from build123d import *

# Parameters (mm, degrees)
SKETCH1_R           = 4.69
SKETCH1_R_2         = 2.2
BOSS_EXTRUDE3_DEPTH = 30
SKETCH3_R           = 4.14334423
SKETCH3_R_2         = 2.739824148
BOSS_EXTRUDE4_DEPTH = 10
SKETCH4_R           = 2.757198723
SKETCH4_R_2         = 1.67402832
BOSS_EXTRUDE5_DEPTH = 10
SKETCH5_R           = 2.2
SKETCH5_R_2         = 1.417715224
BOSS_EXTRUDE6_DEPTH = 10
FILLET13_R          = 5
FILLET15_R          = 5
FILLET16_R          = 5
FILLET17_R          = 5
FILLET19_R          = 5
FILLET20_R          = 5
FILLET21_R          = 5
BOSS_EXTRUDE7_START = -20
SKETCH6_R           = 7.130132291
BOSS_EXTRUDE7_DEPTH = 5
SKETCH7_R           = 3.768659845
CUT_EXTRUDE1_DEPTH  = 30
FILLET26_R          = 5
FILLET27_R          = 5
FILLET28_R          = 5
FILLET29_R          = 5
FILLET30_R          = 5


with BuildPart() as part:
    # Sketch1 → Boss-Extrude3 (new body)
    with BuildSketch(Plane.XY):
        Circle(SKETCH1_R)
        Circle(SKETCH1_R_2, mode=Mode.SUBTRACT)
    extrude(amount=BOSS_EXTRUDE3_DEPTH)

    # Sketch3 → Boss-Extrude4 (add)
    with BuildSketch(Plane.XY.offset(30)):
        Circle(SKETCH3_R)
        Circle(SKETCH3_R_2, mode=Mode.SUBTRACT)
    extrude(amount=BOSS_EXTRUDE4_DEPTH)

    # Sketch4 → Boss-Extrude5 (add)
    with BuildSketch(Plane.XY.offset(40)):
        Circle(SKETCH4_R)
        Circle(SKETCH4_R_2, mode=Mode.SUBTRACT)
    extrude(amount=BOSS_EXTRUDE5_DEPTH)

    # Sketch5 → Boss-Extrude6 (add)
    with BuildSketch(Plane.XY.offset(50)):
        Circle(SKETCH5_R)
        Circle(SKETCH5_R_2, mode=Mode.SUBTRACT)
    extrude(amount=BOSS_EXTRUDE6_DEPTH)

    # Fillet13
    # the kernel refuses this fillet: 5 mm, written as the material it takes off along each edge
    with BuildSketch(Plane(origin=(0, 0, 50), x_dir=(1, 0, 0), z_dir=(0, -1, 0))) as fillet13_piece_1:
        with BuildLine():
            CenterArc((6.417715224, 1.580327356), FILLET13_R, 180, 18.425147301)
            Line((1.417715224, 1.580327356), (1.317715224, 1.580327356))
            Line((1.317715224, 1.580327356), (1.317715224, 0))
            Line((1.317715224, 0), (1.417715224, -0.1))
            ThreePointArc((1.417715224, -0.1), (1.545871772, -0.1), (1.579154581, -0.031606547))
            Line((1.579154581, -0.031606547), (1.67402832, 0))
        make_face()
    revolve(axis=Axis((0, 0, 50), (0, 0, 1)), mode=Mode.SUBTRACT)

    # Fillet15
    fillet15_edges = [part.edges().sort_by_distance(p)[0] for p in [
        (-1.67402832, 0, 50),
    ]]
    fillet(fillet15_edges, radius=FILLET15_R)

    # Fillet16
    # the kernel refuses this fillet: 5 mm, written as the material it adds along each edge
    with BuildSketch(Plane(origin=(0, 0, 50), x_dir=(1, 0, 0), z_dir=(0, -1, 0))) as fillet16_piece_1:
        with BuildLine():
            CenterArc((7.2, 2.293799646), FILLET16_R, 180, 27.307116904)
            Line((2.757198723, 0), (2.668342698, -0.045875993))
            ThreePointArc((2.668342698, -0.045875993), (2.478599362, -0.1), (2.2, -0.1))
            Line((2.2, -0.1), (2.1, 0))
            Line((2.1, 0), (2.1, 2.293799646))
            Line((2.1, 2.293799646), (2.2, 2.293799646))
        make_face()
    revolve(axis=Axis((0, 0, 50), (0, 0, 1)))

    # Fillet17
    # the kernel refuses this fillet: 5 mm, written as the material it takes off along each edge
    with BuildSketch(Plane(origin=(0, 0, 40), x_dir=(1, 0, 0), z_dir=(0, -1, 0))) as fillet17_piece_1:
        with BuildLine():
            CenterArc((6.67402832, 3.085779891), FILLET17_R, 180, 38.108745083)
            Line((2.739824148, 0), (2.661140065, -0.061715598))
            ThreePointArc((2.661140065, -0.061715598), (2.206926234, -0.1), (1.67402832, -0.1))
            Line((1.67402832, -0.1), (1.57402832, 0))
            Line((1.57402832, 0), (1.57402832, 3.085779891))
            Line((1.57402832, 3.085779891), (1.67402832, 3.085779891))
        make_face()
    revolve(axis=Axis((0, 0, 40), (0, 0, 1)), mode=Mode.SUBTRACT)

    # Fillet18: read off the stored shape, not the designer's step
    # Fillet18 outline → Fillet18 (revolve)
    with BuildSketch(Plane.XZ):
        with BuildLine():
            Line((2.757198723, 40), (4.14334423, 40))
            ThreePointArc((4.14334423, 40), (3.116656057, 41.593889814), (2.757198723, 43.455438569))
            Line((2.757198723, 43.455438569), (2.757198723, 40))
        make_face()
    revolve(axis=Axis((0, 0, 0), (0, 0, 1)))

    # Fillet19
    fillet19_edges = [part.edges().sort_by_distance(p)[0] for p in [
        (-2.739824148, 0, 40),
    ]]
    fillet(fillet19_edges, radius=FILLET19_R)

    # Fillet20
    fillet20_edges = [part.edges().sort_by_distance(p)[0] for p in [
        (-4.14334423, 0, 40),
    ]]
    fillet(fillet20_edges, radius=FILLET20_R)

    # Fillet21
    # the kernel refuses this fillet: 5 mm, written as the material it adds along each edge
    with BuildSketch(Plane(origin=(0, 0, 30), x_dir=(1, 0, 0), z_dir=(0, -1, 0))) as fillet21_piece_1:
        with BuildLine():
            CenterArc((9.14334423, 2.27326311), FILLET21_R, 180, 27.042585546)
            Line((4.69, 0), (4.600933115, -0.045465262))
            ThreePointArc((4.600933115, -0.045465262), (4.416672115, -0.1), (4.14334423, -0.1))
            Line((4.14334423, -0.1), (4.04334423, 0))
            Line((4.04334423, 0), (4.04334423, 2.27326311))
            Line((4.04334423, 2.27326311), (4.14334423, 2.27326311))
        make_face()
    revolve(axis=Axis((0, 0, 30), (0, 0, 1)))

    # Sketch6 → Boss-Extrude7 (add)
    with BuildSketch(Plane(origin=(0, 0, 0), x_dir=(-1, 0, 0), z_dir=(0, 0, -1)).offset(BOSS_EXTRUDE7_START)):
        Circle(SKETCH6_R)
    extrude(amount=BOSS_EXTRUDE7_DEPTH)

    # Sketch7 → Cut-Extrude1 (cut)
    with BuildSketch(Plane(origin=(0, 0, 0), x_dir=(-1, 0, 0), z_dir=(0, 0, -1))):
        Circle(SKETCH7_R)
    extrude(amount=-CUT_EXTRUDE1_DEPTH, mode=Mode.SUBTRACT)

    # Fillet26
    # the kernel refuses this fillet: 5 mm, written as the material it adds along each edge
    with BuildSketch(Plane(origin=(0, 0, 20), x_dir=(1, 0, 0), z_dir=(0, 1, 0))) as fillet26_piece_1:
        with BuildLine():
            CenterArc((9.69, -4.29500609), FILLET26_R, 120.795376003, 59.204623997)
            Line((7.130132291, 0), (7.078934937, 0.085900122))
            ThreePointArc((7.078934937, 0.085900122), (5.910066146, 0.1), (4.69, 0.1))
            Line((4.69, 0.1), (4.59, 0))
            Line((4.59, 0), (4.59, -4.29500609))
            Line((4.59, -4.29500609), (4.69, -4.29500609))
        make_face()
    revolve(axis=Axis((0, 0, 20), (0, 0, -1)))

    # Fillet27
    # the kernel refuses this fillet: 5 mm, written as the material it takes off along each edge
    with BuildSketch(Plane(origin=(0, 0, 15), x_dir=(-1, 0, 0), z_dir=(0, -1, 0))) as fillet27_piece_1_section:
        with BuildLine():
            CenterArc((2.130132291, -4.29500609), FILLET27_R, 0, 59.204623997)
            Line((4.69, 0), (4.741197354, 0.085900122))
            ThreePointArc((4.741197354, 0.085900122), (5.910066146, 0.1), (7.130132291, 0.1))
            Line((7.130132291, 0.1), (7.230132291, 0))
            Line((7.230132291, 0), (7.230132291, -4.29500609))
            Line((7.230132291, -4.29500609), (7.130132291, -4.29500609))
        make_face()
    fillet27_piece_1 = revolve(axis=Axis((0, 0, 15), (0, 0, -1)), mode=Mode.PRIVATE)
    fillet27_piece_1 = fillet27_piece_1 - Plane(origin=(0, 0, 15), x_dir=(1, 0, 0), z_dir=(0, 0, -1)) * Cylinder(4.69, 29, mode=Mode.PRIVATE)
    add(fillet27_piece_1, mode=Mode.SUBTRACT)

    # Fillet28
    # the kernel refuses this fillet: 5 mm, written as the material it adds along each edge
    with BuildSketch(Plane(origin=(0, 0, 15), x_dir=(-1, 0, 0), z_dir=(0, -1, 0))) as fillet28_piece_1:
        with BuildLine():
            CenterArc((9.69, 2.250862854), FILLET28_R, 180, 40.888333518)
            Line((4.69, 2.250862854), (4.69, 0))
            ThreePointArc((4.69, 0), (5.340962178, -0.462177965), (5.910066146, -1.022071618))
        make_face()
    revolve(axis=Axis((0, 0, 15), (0, 0, -1)), revolution_arc=180)
    with BuildSketch(Plane(origin=(0, 0, 15), x_dir=(1, 0, 0), z_dir=(0, 1, 0))) as fillet28_piece_2:
        with BuildLine():
            CenterArc((9.69, 2.250862854), FILLET28_R, 180, 40.888333518)
            Line((4.69, 2.250862854), (4.69, 0))
            ThreePointArc((4.69, 0), (5.340962178, -0.462177965), (5.910066146, -1.022071618))
        make_face()
    revolve(axis=Axis((0, 0, 15), (0, 0, -1)), revolution_arc=180)
    # the kernel refuses this fillet: 5 mm, written as the material it takes off along each edge
    with BuildSketch(Plane(origin=(0, 0, 20), x_dir=(-1, 0, 0), z_dir=(0, -1, 0))) as fillet28_2_piece_1:
        with BuildLine():
            CenterArc((2.546742384, 2.703127277), FILLET28_R, 315.587970102, 20.857187789)
            Line((7.130132291, 0.70499391), (7.130132291, 0))
            ThreePointArc((7.130132291, 0), (6.598529109, -0.365272291), (6.118371192, -0.795939407))
        make_face()
    revolve(axis=Axis((0, 0, 20), (0, 0, -1)), revolution_arc=180, mode=Mode.SUBTRACT)
    with BuildSketch(Plane(origin=(0, 0, 20), x_dir=(1, 0, 0), z_dir=(0, 1, 0))) as fillet28_2_piece_2:
        with BuildLine():
            CenterArc((2.546742384, 2.703127277), FILLET28_R, 315.587970102, 20.857187789)
            Line((7.130132291, 0.70499391), (7.130132291, 0))
            ThreePointArc((7.130132291, 0), (6.598529109, -0.365272291), (6.118371192, -0.795939407))
        make_face()
    revolve(axis=Axis((0, 0, 20), (0, 0, -1)), revolution_arc=180, mode=Mode.SUBTRACT)

    # Fillet29
    # the kernel refuses this fillet: 5 mm, written as the material it takes off along each edge
    with BuildSketch(Plane(origin=(0, 0, 30), x_dir=(1, 0, 0), z_dir=(0, -1, 0))) as fillet29_piece_1:
        with BuildLine():
            CenterArc((7.739824148, 3.038067491), FILLET29_R, 180, 37.417142661)
            Line((2.739824148, 3.038067491), (2.639824148, 3.038067491))
            Line((2.639824148, 3.038067491), (2.639824148, 0))
            Line((2.639824148, 0), (2.739824148, -0.1))
            ThreePointArc((2.739824148, -0.1), (3.254241996, -0.1), (3.689236559, -0.06076135))
            Line((3.689236559, -0.06076135), (3.768659845, 0))
        make_face()
    revolve(axis=Axis((0, 0, 30), (0, 0, 1)), mode=Mode.SUBTRACT)

    # Fillet30
    fillet30_edges = [part.edges().sort_by_distance(p)[0] for p in [
        (0, -3.768659845, 30),
    ]]
    fillet(fillet30_edges, radius=FILLET30_R)


solid = part.part
Source: CAD feature listing. Evaluate the final solid. Frame: model axes, mm. A direction names the side the tool comes from. Give positions to 0.01 mm unless a question says otherwise; leave off trailing zeros. Write each loop counter-clockwise with the first axis right and the second up, starting at its lowest first coordinate (ties: lowest second). Pieces come first, ordered by that corner, then holes. Notation, with made-up numbers: (26, -27.5) -> (63, -27.5) arc R16 cw to (63, -23.5) -> close; hole circle Ø1 at (-37, 68). An arc over 180 degrees is marked (long way). Write item = value, one per line.
Q1. Reachability of faces 4 (the face through (-0.307, -1.384, 55.731)), 5 (the face through (2.613, 0.823, 35.777)), 6 (the face through (-2, 1.9, 46.7)) from +Z, -Z, +X, -X, +Y, -Y: full face, straight path, thin tool, end or side. Return the list, or none.
Here are the results:
face_4 = +Z, -Z
face_5 = -Z
face_6 = +Z
Q2. Cut plane A-A on z = 14.5. Return loops of the section in (x, y).
Here are the results:
outline = circle Ø10.01 at (0, 0); hole circle Ø7.54 at (0, 0)
Q3. Mould query, pull axis X, two halves, no side actions, for faces 1 (the face through (-3.595, 1.132, 14.112)), 2 (the face through (2.1, 0.66, 56.09)), 3 (the face through (0, 4, 0)). Classes: +X half, -X half, draft (parallel to the pull), parting line (faces both ways), or undercut.
Here are the results:
face_1 = undercut
face_2 = parting line
face_3 = draft
Q4. First-contact query: pin 1 (5 mm diameter, centred on y = -0.5, z = 34, fed in from +X); pin 2 (2.5 mm diameter, centred on x = 0, y = 0, fed in from -Z); pin 3 (1.5 mm diameter, centred on x = 0.5, z = 52.5, fed in from +Y); pin 4 (4.5 mm diameter, centred on x = 0, y = 0, fed in from -Z). Flat tips, straight axial feed; report the tip coordinate or a pass-through.
Here are the results:
pin_1 = 4.2
pin_2 = through
pin_3 = 2.22
pin_4 = 40.75
Q5. Line query: line 1 (Y direction, x = 0, z = 47.5); line 2 (Y direction, x = 0, z = 37.1); line 3 (X direction, y = 1, z = 37). Output: solid intervals per line, ascending. Write a range as from..to.
Here are the results:
line_1 = -2.76..-1.67, 1.67..2.76
line_2 = -4.14..-2.74, 2.74..4.14
line_3 = -4.02..-2.55, 2.55..4.02
